CAD build for the part. Positions are in the model's coordinates, mm. A direction names the side the tool comes from. Round coordinates to 2 decimals unless told otherwise and drop trailing zeros. Loops run counter-clockwise (first coordinate to the right, second up) from the corner with the lowest first, then second, coordinate; pieces in that order, holes last.
```python
from build123d import *

# Parameters (mm, degrees)
F0_W     = 60.4
F0_H     = 42
F1_DEPTH = 21.2
F2_R     = 2
F3_R     = 9
F3_R_2   = 12.25
F4_DEPTH = 0.5
F3_R_3   = 8
F5_DEPTH = 0.5
F6_DEPTH = 7.5
F10_R    = 1.5
F11_R    = 0.49999
F12_R    = 0.49999


# Not quite as in the source:
# - a fillet or chamfer is up to 0.001 mm smaller than in the source, because OpenCascade refuses the exact size


with BuildPart() as f1:
    # F0 (on Front) → F1 (new body)
    with BuildSketch(Plane.XZ):
        with Locations((0, 21)):
            Rectangle(F0_W, F0_H)
    extrude(amount=F1_DEPTH)

    # F2
    f2_edges = [f1.edges().sort_by_distance(p)[0] for p in [
        (-30.2, -10.6, 42),
        (30.2, -10.6, 42),
        (30.2, -10.6, 0),
        (-30.2, -10.6, 0),
    ]]
    fillet(f2_edges, radius=F2_R)

    # F3 (on face) → F4 (cut)
    with BuildSketch(Plane.XZ.offset(21.2)):
        with BuildLine():
            ThreePointArc((2.9912166904, 9.75), (3.1651187763, 9.7187836009), (3.3173064746, 9.6290322581))
            ThreePointArc((3.3173064746, 9.6290322581), (28.1, 21), (3.3173064746, 32.3709677419))
            ThreePointArc((3.3173064746, 32.3709677419), (3.1651187763, 32.2812163991), (2.9912166904, 32.25))
            Line((2.9912166904, 32.25), (-15.4, 32.25))
            ThreePointArc((-15.4, 32.25), (-26.65, 21), (-15.4, 9.75))
            Line((-15.4, 9.75), (2.9912166904, 9.75))
        make_face()
        with Locations((-15.4, 21)):
            Circle(F3_R, mode=Mode.SUBTRACT)
        with Locations((13.1, 21)):
            Circle(F3_R_2, mode=Mode.SUBTRACT)
    extrude(amount=-F4_DEPTH, mode=Mode.SUBTRACT)

    # F3 (on face) → F5 (cut)
    with BuildSketch(Plane.XZ.offset(21.2)):
        with Locations((-15.4, 21)):
            Circle(F3_R_3)
    extrude(amount=-F5_DEPTH, mode=Mode.SUBTRACT)

    # F3 (on face) → F6 (join)
    with BuildSketch(Plane.XZ.offset(21.2)):
        with Locations((13.1, 21)):
            Circle(F3_R_2)
    extrude(amount=F6_DEPTH)

    # F8 (on offset) → F9 (revolve, cut)
    with BuildSketch(Plane.YZ.offset(13.1)):
        with BuildLine():
            ThreePointArc((-28.2, 21), (-27.6105631935, 25.1636124275), (-25.8885775404, 29))
            Line((-25.8885775404, 29), (-28.7, 29))
            Line((-28.7, 29), (-28.7, 21))
            Line((-28.7, 21), (-28.2, 21))
        make_face()
    revolve(axis=Axis((13.1, -14.35, 21), (0, 1, 0)), mode=Mode.SUBTRACT)

    # F10
    f10_edges = [f1.edges().sort_by_distance(p)[0] for p in [
        (0.85, -20.7, 21),
    ]]
    fillet(f10_edges, radius=F10_R)

    # F11 (radius 0.5 in the source; OpenCascade refuses exactly that, so slightly less here)
    f11_edges = [f1.edges().sort_by_distance(p)[0] for p in [
        (-0.65, -20.7, 21),
        (-6.204392, -20.7, 9.75),
        (3.165119, -20.7, 9.718784),
        (28.1, -20.7, 21),
        (3.165119, -20.7, 32.281216),
        (-6.204392, -20.7, 32.25),
        (-26.65, -20.7, 21),
        (-24.4, -20.7, 21),
    ]]
    fillet(f11_edges, radius=F11_R)

    # F12 (radius 0.5 in the source; OpenCascade refuses exactly that, so slightly less here)
    f12_edges = [f1.edges().sort_by_distance(p)[0] for p in [
        (-23.4, -20.7, 21),
    ]]
    fillet(f12_edges, radius=F12_R)


solid = f1.part
```
Item 1: Cut at A-A, the plane y = -27. Give the cut face in (x, z), plus the area to 3 significant figures.
Answers follow:
outline: circle Ø24.5 at (13.1, 21); circle Ø11.76 at (13.1, 21); hole circle Ø16 at (13.1, 21)
area: 379 mm2
Item 2: 3-axis set-ups, long thin cutter, end or side, ignore diameter. For faces 5 (the flat face through (-21, -21.2, 15)), 6 (the cylindrical face through (3.379, -25.404, 13.546)), 7 (the cylindrical face through (-29.63, -10.75, 0.6)): which of +Z, -Z, +X, -X, +Y, -Y reach the whole face in a straight line?
Answers follow:
face 5: +Z, -Z, -X, -Y
face 6: -Y
face 7: -Z, -X, +Y, -Y
Item 3: Two-plate mould, pull along Z, no slides. Class faces 1 (the flat face through (0, -10, 42)), 2 (the flat face through (-3, -20.7, 20)), 3 (the flat face through (-16, -20.7, 21)), 4 (the flat face through (30.2, -10, 21)): released by +Z, released by -Z, zero draft, split by the parting line, or undercut.
Answers follow:
face 1: released by +Z
face 2: undercut
face 3: undercut
face 4: zero draft
Item 4: Probe line 1 (X direction, y = -26.7, z = 21); line 2 (Y direction, x = 15.5, z = 7.5); line 3 (Y direction, x = -13.5, z = 5). List the from-to ranges inside material, lowest first.
Answers follow:
line 1: x = 0.85 to 5.1, 6.56 to 19.64, 21.1 to 25.35
line 2: y = -20.7 to 0
line 3: y = -21.2 to 0
Item 5: Flat gauge pins, fed straight in: P1, Ø14.5, axis at x = -15.4, z = 21, coming from the -Y side; P2, Ø13, axis at x = 13.1, z = 21, coming from the -Y side. Where does each tip first touch, or does it go through?
Answers follow:
P1: stops at y = -20.7
P2: stops at y = -28.2
Item 6: Cut at B-B, the plane z = 37. Give the cut face in (x, y).
Answers follow:
outline: (-30.2, -21.2) - (30.2, -21.2) - (30.2, 0) - (-30.2, 0) - close
